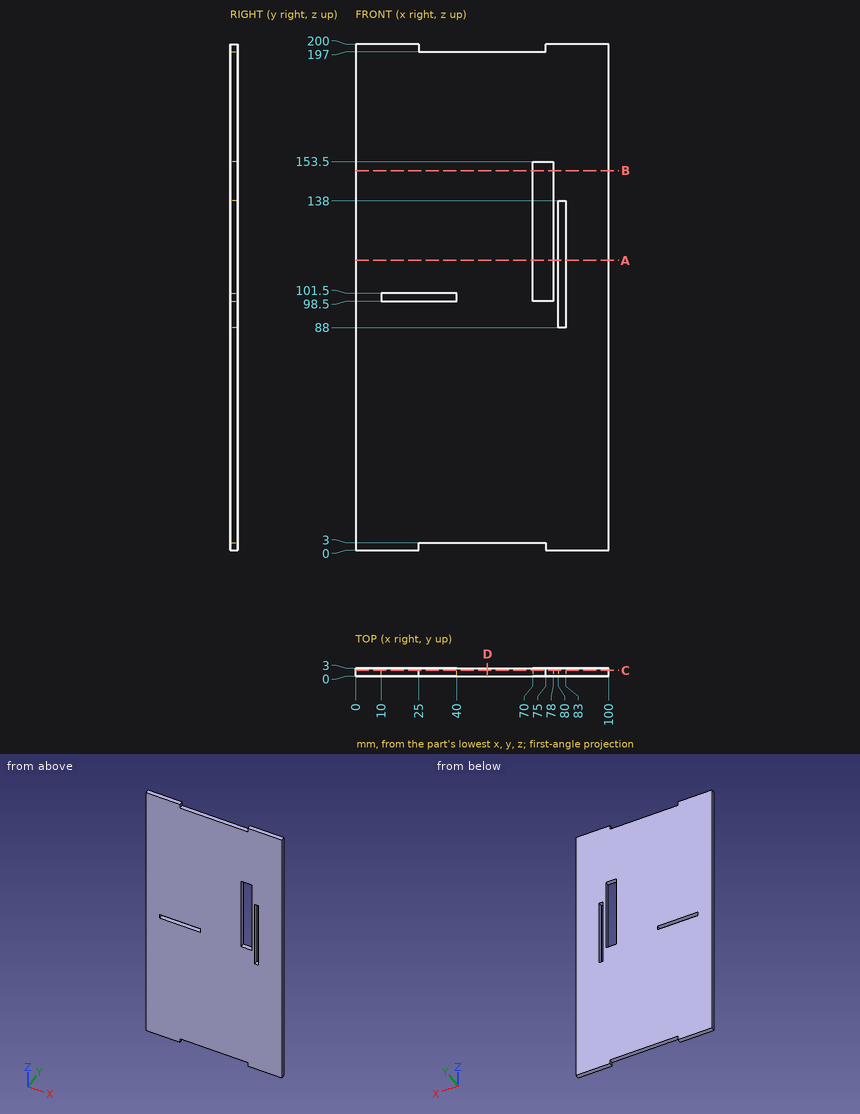
Verification items for this drawing (mm, ordinates from the low corner). Round coordinates to 2 decimals unless told otherwise and drop trailing zeros. Write each loop counter-clockwise with the first axis right and the second up, starting at its lowest first coordinate (ties: lowest second). Pieces come first, ordered by that corner, then holes. Notation, with made-up numbers: (71, 45.5) - (120, 45.5) arc R14 cw to (120, 60.5) - close; hole circle Ø9 at (32, 18.25). An arc over 180 degrees is marked (long way). One line per item, written item: value.
1. Depth check by flat-ended pin: pin 1 Ø1 at (x, y) = (60, 2) entering from -Z; pin 2 Ø1.5 at (x, y) = (52, 1) entering from +Z. Enter the tip coordinate at first touch or a pass-through.
The answers:
pin 1: stops at z = 3
pin 2: stops at z = 197
2. Scan lines: L1, parallel to X at y = 0.2, z = 109.5; L2, parallel to Z at x = 16, y = 1.4; L3, parallel to Z at x = 37, y = 0.75. Record each from-to range of solid material in increasing order.
The answers:
L1: x = 0 to 70, 78 to 80, 83 to 100
L2: z = 0 to 98.5, 101.5 to 200
L3: z = 3 to 98.5, 101.5 to 197
3. Cross-section at C-C on y = 2.25. Record the boundary of the cut face in (x, z), and give its area (3 significant figures).
The answers:
outline: (0, 0) - (25, 0) - (25, 3) - (75, 3) - (75, 0) - (100, 0) - (100, 200) - (75, 200) - (75, 197) - (25, 197) - (25, 200) - (0, 200) - close; hole (10, 98.5) - (40, 98.5) - (40, 101.5) - (10, 101.5) - close; hole (70, 98.5) - (78, 98.5) - (78, 153.5) - (70, 153.5) - close; hole (80, 88) - (83, 88) - (83, 138) - (80, 138) - close
area: 19,000 mm^2
4. Cross-section at B-B on z = 150. Record the boundary of the cut face in (x, y), and give its area (3 significant figures).
The answers:
outline: (0, 0) - (70, 0) - (70, 3) - (0, 3) - close; (78, 0) - (100, 0) - (100, 3) - (78, 3) - close
area: 276 mm^2
5. Cross-section at A-A on z = 114.5. Record the boundary of the cut face in (x, y), and give its area (3 significant figures).
The answers:
outline: (0, 0) - (70, 0) - (70, 3) - (0, 3) - close; (78, 0) - (80, 0) - (80, 3) - (78, 3) - close; (83, 0) - (100, 0) - (100, 3) - (83, 3) - close
area: 267 mm^2
6. Cross-section at D-D on x = 52. Record the boundary of the cut face in (y, z), and give its area (3 significant figures).
The answers:
outline: (0, 3) - (3, 3) - (3, 197) - (0, 197) - close
area: 582 mm^2
